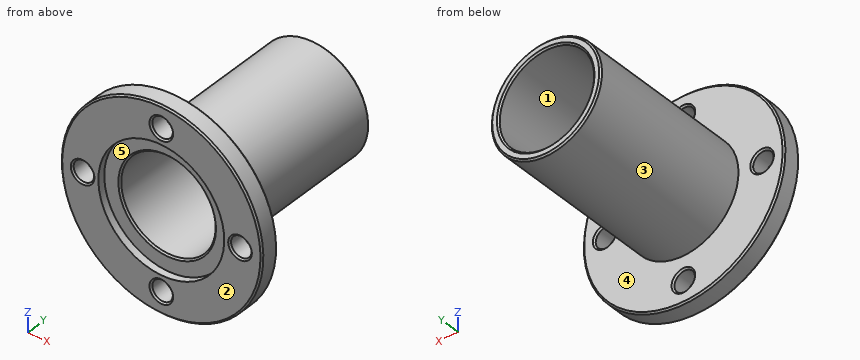
```python
from build123d import *

# Parameters (mm, degrees)
SKETCH1_R           = 32
BOSS_EXTRUDE1_DEPTH = 60
SKETCH2_OUTSIDE_W   = 87.718
SKETCH2_OUTSIDE_H   = 87.718
SKETCH2_OUTSIDE_R   = 17.5
CUT_EXTRUDE1_DEPTH  = 54
SKETCH4_R           = 20
CUT_EXTRUDE2_DEPTH  = 2.3
SKETCH5_R           = 15
CUT_EXTRUDE3_DEPTH  = 74.3300075
CHAMFER1_SIZE       = 0.5
SKETCH6_R           = 3.25
CUT_EXTRUDE4_DEPTH  = 76.153176912
CHAMFER2_SIZE       = 0.5


with BuildPart() as part:
    # Sketch1 → Boss-Extrude1 (new body)
    with BuildSketch(Plane(origin=(0, 0, 0), x_dir=(1, 0, 0), z_dir=(0, 1, 0))):
        with Locations(Location((0, 0, 0), (0, 0, 270))):
            Circle(SKETCH1_R)
    extrude(amount=BOSS_EXTRUDE1_DEPTH)

    # Sketch2 outside → Cut-Extrude1 (cut)
    with BuildSketch(Plane(origin=(0, 60, 0), x_dir=(1, 0, 0), z_dir=(0, 1, 0))):
        Rectangle(SKETCH2_OUTSIDE_W, SKETCH2_OUTSIDE_H)
        with Locations(Location((0, 0, 0), (0, 0, 270))):
            Circle(SKETCH2_OUTSIDE_R, mode=Mode.SUBTRACT)
    extrude(amount=-CUT_EXTRUDE1_DEPTH, mode=Mode.SUBTRACT)

    # Sketch4 → Cut-Extrude2 (cut)
    with BuildSketch(Plane.XZ):
        with Locations(Location((0, 0, 0), (0, 0, 270))):
            Circle(SKETCH4_R)
    extrude(amount=-CUT_EXTRUDE2_DEPTH, mode=Mode.SUBTRACT)

    # Sketch5 → Cut-Extrude3 (cut, through all)
    with BuildSketch(Plane.XZ.offset(-2.3)):
        with Locations(Location((0, 0, 0), (0, 0, 270))):
            Circle(SKETCH5_R)
    extrude(amount=-CUT_EXTRUDE3_DEPTH, mode=Mode.SUBTRACT)

    # Chamfer1
    chamfer1_edges = [part.edges().sort_by_distance(p)[0] for p in [
        (0, 60, -17.5),
        (0, 0, -32),
        (0, 60, 15),
        (0, 2.3, 15),
        (0, 6, -32),
    ]]
    chamfer(chamfer1_edges, length=CHAMFER1_SIZE)

    # Sketch6 → Cut-Extrude4 (cut, through all)
    with BuildSketch(Plane.XZ):
        with Locations(Location((25, 0, 0), (0, 0, 270))):
            Circle(SKETCH6_R)
        with Locations(Location((0, -25, 0), (0, 0, 270))):
            Circle(SKETCH6_R)
        with Locations(Location((-25, 0, 0), (0, 0, 270))):
            Circle(SKETCH6_R)
        with Locations(Location((0, 25, 0), (0, 0, 270))):
            Circle(SKETCH6_R)
    extrude(amount=-CUT_EXTRUDE4_DEPTH, mode=Mode.SUBTRACT)

    # Chamfer2
    chamfer2_edges = [part.edges().sort_by_distance(p)[0] for p in [
        (25, 6, 3.25),
        (25, 0, 3.25),
        (0, 6, -21.75),
        (0, 0, -21.75),
        (-25, 6, 3.25),
        (-25, 0, 3.25),
        (0, 6, 28.25),
        (0, 0, 28.25),
    ]]
    chamfer(chamfer2_edges, length=CHAMFER2_SIZE)


solid = part.part
```
Could you check a few things on this model? Use its own coordinates, in mm. Face numbers are marked on the shaded views. A direction names the side the tool comes from. Coordinates: 2 decimals unless noted, no trailing zeros. Loops run counter-clockwise (first coordinate to the right, second up) from the corner with the lowest first, then second, coordinate; pieces in that order, holes last.
1) Thinking about a two-plate mould opening in Z: for the marked faces 1, 2 and 3, which applies, released by +Z, released by -Z, zero draft, split by the parting line, or undercut?
Reported:
face 1: undercut
face 2: zero draft
face 3: split by the parting line
2) Please list where these lines run through material, in increasing order: line 1 along X through (y, z) = (1, 0); line 2 along X through (y, z) = (43, 0); line 3 along X through (y, z) = (4.2, 0).
Reported:
line 1: x = -32 to -28.25, -21.75 to -20, 20 to 21.75, 28.25 to 32
line 2: x = -17.5 to -15, 15 to 17.5
line 3: x = -32 to -28.25, -21.75 to -15, 15 to 21.75, 28.25 to 32
3) Imagine slicing it at B-B (y = 26.5). List the corners of the cut face in (x, z) for me, and give its area (3 significant figures).
Reported:
outline: circle Ø35 at (0, 0); hole circle Ø30 at (0, 0)
area: 255 mm2
4) Which directions (+Z, -Z, +X, -X, +Y, -Y) give clear straight access to the entire face, cutting with the end or side of a thin tool? Please do the marked faces 4 and 5.
Reported:
face 4: +Y
face 5: -Y
5) Imagine slicing it at A-A (x = 0). State how many separate pieces and enclosed holes the cut face has, and give its area (3 significant figures).
Reported:
separate pieces: 4
enclosed holes: 0
area: 371 mm2
6) Will these pins go through, and if not, where does the flat tip stop? pin 1 Ø10 at (x, y) = (19.5, 25.5) entering from -Z; pin 2 Ø1 at (x, z) = (14, 17) entering from -Y; pin 3 Ø8.5 at (x, z) = (25, 0) entering from +Y; pin 4 Ø12 at (x, y) = (11.5, 41) entering from -Z.
Reported:
pin 1: stops at z = -9.8
pin 2: stops at y = 0
pin 3: stops at y = 6
pin 4: stops at z = -16.61
